Input: part model. Units: mm. Frame: model coordinates. Face numbers are marked on the shaded views. A direction names the side the tool comes from. Give positions to 0.01 mm unless a question says otherwise; leave off trailing zeros. Loops run counter-clockwise (first coordinate to the right, second up) from the corner with the lowest first, then second, coordinate; pieces in that order, holes last. Notation, with made-up numbers: (9, 69.5) - (32, 69.5) arc R23 cw to (32, 99.5) - close; hole circle Ø3 at (-33, -22.75). An arc over 180 degrees is marked (long way). One line per item, written item: value.
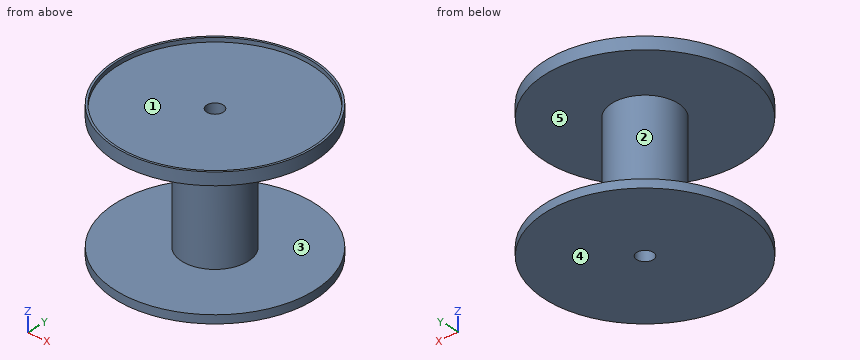
from build123d import *

# Parameters (mm, degrees)
F0_R     = 152.4
F1_DEPTH = 12.7
F2_R     = 50.8
F3_DEPTH = 177.8
F4_R     = 152.4
F4_R_2   = 50.8
F5_DEPTH = 12.7
F6_R     = 152.4
F6_R_2   = 149.225
F7_DEPTH = 6.35
F8_R     = 12.7
F9_DEPTH = 457.2


with BuildPart() as f1:
    # F0 (on Top) → F1 (new body)
    with BuildSketch(Plane.XY):
        Circle(F0_R)
    extrude(amount=F1_DEPTH)

    # F2 (on face) → F3 (join)
    with BuildSketch(Plane.XY.offset(12.7)):
        Circle(F2_R)
    extrude(amount=F3_DEPTH)

    # F4 (on face) → F5 (join)
    with BuildSketch(Plane.XY.offset(190.5)):
        Circle(F4_R)
        Circle(F4_R_2, mode=Mode.SUBTRACT)
        Circle(F4_R_2)
    extrude(amount=F5_DEPTH)

    # F6 (on face) → F7 (join)
    with BuildSketch(Plane.XY.offset(203.2)):
        Circle(F6_R)
        Circle(F6_R_2, mode=Mode.SUBTRACT)
    extrude(amount=F7_DEPTH)

    # F8 (on face) → F9 (cut)
    with BuildSketch(Plane.XY.offset(203.2)):
        Circle(F8_R)
    extrude(amount=-F9_DEPTH, mode=Mode.SUBTRACT)


solid = f1.part
Item 1: Section A-A, the plane y = 0. Output: boundary loops of the cut face in (x, z) (3 decimals), and give its area (3 significant figures).
Verdict:
outline: (-152.4, 0) - (-12.7, 0) - (-12.7, 203.2) - (-149.225, 203.2) - (-149.225, 209.55) - (-152.4, 209.55) - (-152.4, 190.5) - (-50.8, 190.5) - (-50.8, 12.7) - (-152.4, 12.7) - close; (12.7, 0) - (152.4, 0) - (152.4, 12.7) - (50.8, 12.7) - (50.8, 190.5) - (152.4, 190.5) - (152.4, 209.55) - (149.225, 209.55) - (149.225, 203.2) - (12.7, 203.2) - close
area: 20,700 mm^2
Item 2: Draft query along X for the marked faces 1, 2 and 3. Return one class per face: pulls with the +X half, pulls with the -X half, needs draft (parallel to the pull), parting line crosses it, or undercut.
Verdict:
face 1: undercut
face 2: parting line crosses it
face 3: needs draft
Item 3: Section C-C, the plane z = 155. Output: boundary loops of the cut face in (x, y), and give its area (3 significant figures).
Verdict:
outline: circle Ø101.6 at (0, 0); hole circle Ø25.4 at (0, 0)
area: 7,600 mm^2
Item 4: Access query for the marked faces 4 and 5. Directions: +Z, -Z, +X, -X, +Y, -Y. A direction counts if a zero-diameter tool reaches every point of the face in a straight line with its end or side. Return the directions, or none.
Verdict:
face 4: -Z, +X, -X, +Y, -Y
face 5: none
Item 5: Pin query (flat end, axial travel): P1, Ø4, axis at x = 19.5, y = 95, coming from the -Z side; P2, Ø3, axis at x = -47.5, y = -3.5, coming from the +Z side; P3, Ø1, axis at y = -46.5, z = 104.5, coming from the +X side. Return the tip coordinate at first contact, or that it passes through.
Verdict:
P1: stops at z = 0
P2: stops at z = 203.2
P3: stops at x = 21.56
Item 6: Material intervals for L1, parallel to Z at x = -42.5, y = 131.5; L2, parallel to Y at x = 0, z = 111; L3, parallel to Y at x = 0, z = 204 (3 decimals), sorted ascending.
Verdict:
L1: z = 0 to 12.7, 190.5 to 203.2
L2: y = -50.8 to -12.7, 12.7 to 50.8
L3: y = -152.4 to -149.225, 149.225 to 152.4
Item 7: Section D-D, the plane y = 123. Output: boundary loops of the cut face in (x, z), and give its area (3 significant figures).
Verdict:
outline: (-89.98, 0) - (89.98, 0) - (89.98, 12.7) - (-89.98, 12.7) - close; (-89.98, 190.5) - (89.98, 190.5) - (89.98, 209.55) - (84.49, 209.55) - (84.49, 203.2) - (-84.49, 203.2) - (-84.49, 209.55) - (-89.98, 209.55) - close
area: 4,640 mm^2
